```python
from build123d import *

# Parameters (mm, degrees)
ESQUISSE1_R          = 0.6
BASE_EXTRUSION_DEPTH = 1


with BuildPart() as part:
    # Esquisse1 → Base-Extrusion (new body)
    with BuildSketch(Plane.XY):
        with BuildLine():
            Line((-4.406978672, 11.661475663), (-4.564568548, 12.078480291))
            ThreePointArc((-4.564568548, 12.078480291), (-5.131923481, 12.654767663), (-5.94, 12.622969933))
            ThreePointArc((-5.94, 12.622969933), (0, -13), (5.94, 12.622969933))
            ThreePointArc((5.94, 12.622969933), (5.131923481, 12.654767663), (4.564568548, 12.078480291))
            Line((4.564568548, 12.078480291), (4.406978672, 11.661475663))
            ThreePointArc((4.406978672, 11.661475663), (2.882284348, 12.148709668), (1.306307585, 12.428686453))
            Line((1.306307585, 12.428686453), (1.567926949, 14.917828431))
            ThreePointArc((1.567926949, 14.917828431), (0, -15), (-1.567926949, 14.917828431))
            Line((-1.567926949, 14.917828431), (-1.306307585, 12.428686453))
            ThreePointArc((-1.306307585, 12.428686453), (-2.882284348, 12.148709668), (-4.406978672, 11.661475663))
        make_face()
        with Locations((-3, 13.4)):
            Circle(ESQUISSE1_R, mode=Mode.SUBTRACT)
        with Locations(Location((3, 13.4, 0), (0, 0, 180))):
            Circle(ESQUISSE1_R, mode=Mode.SUBTRACT)
    extrude(amount=BASE_EXTRUSION_DEPTH)


solid = part.part
```
Check sheet for the modelled part. Datum: model origin and axes. Units: mm. A direction names the side the tool comes from. Coordinates: 2 decimals unless noted, no trailing zeros. Loops run counter-clockwise (first coordinate to the right, second up) from the corner with the lowest first, then second, coordinate; pieces in that order, holes last.
1) Release check for a two-part mould opening along X. For faces 4 (the face through (5.14, 12.66, 0.49)), 5 (the face through (0.1, -13.3, 1)), 6 (the face through (0.638, -14.986, 0.493)) record: released by +X, released by -X, zero draft, split by the parting line, or undercut.
2) Sectioned sample at D-D (x = -9.5). Record the boundary of the cut face in (y, z), and give its area (3 significant figures).
3) Sectioned sample at C-C (x = 3). Record the boundary of the cut face in (y, z), and give its area (3 significant figures).
4) Access from +Z, -Z, +X, -X, +Y, -Y to the whole of each face (thin tool, end or side, straight path). Record for faces 1 (the face through (1.435, 13.656, 0.493)), 2 (the face through (0.1, -13.3, 0)), 3 (the face through (2.904, 12.143, 0.493)).
5) Sectioned sample at B-B (y = 8.25). Record the boundary of the cut face in (x, z).
6) Sectioned sample at A-A (z = 0.5). Record the boundary of the cut face in (x, y), and give its area (3 significant figures).
7) Gauge pin test, flat end, axial feed: pin 1 (1.4 mm diameter, centred on x = 3, y = 13.4, fed in from +Z). Record the tip position at first contact, or that the pin passes through.
8) Material ranges on probe 1 along Y at (x, z) = (3, 0.6); probe 2 along Y at (x, z) = (3.5, 0.15); probe 3 along X at (y, z) = (0.5, 0.65), recorded low to high.
Check sheet entries:
1. face 4: undercut
1. face 5: zero draft
1. face 6: split by the parting line
2. outline: (-11.61, 0) - (-9.09, 0) - (-9.09, 1) - (-11.61, 1) - close; (10.09, 0) - (11.61, 0) - (11.61, 1) - (10.09, 1) - close
2. area: 4.03 mm2
3. outline: (-14.7, 0) - (-12.66, 0) - (-12.66, 1) - (-14.7, 1) - close; (12.12, 0) - (12.8, 0) - (12.8, 1) - (12.12, 1) - close; (14, 0) - (14.7, 0) - (14.7, 1) - (14, 1) - close
3. area: 3.41 mm2
4. face 1: +Z, -Z, +Y
4. face 2: -Z, +X, -X, +Y, -Y
4. face 3: +Z, -Z
5. outline: (-12.53, 0) - (-11.05, 0) - (-11.05, 1) - (-12.53, 1) - close; (11.05, 0) - (12.53, 0) - (12.53, 1) - (11.05, 1) - close
6. outline: (-5.94, 12.62) arc R1 cw to (-4.56, 12.08) - (-4.41, 11.66) arc R12 cw to (-1.31, 12.43) - (-1.57, 14.92) arc R15 ccw (long way) to (1.57, 14.92) - (1.31, 12.43) arc R12 cw to (4.41, 11.66) - (4.56, 12.08) arc R1 cw to (5.94, 12.62) arc R13.5 cw (long way) to start; hole circle Ø1.2 at (-3, 13.4); hole circle Ø1.2 at (3, 13.4)
6. area: 140 mm2
7. pin 1: stops at z = 1
8. probe 1: y = -14.7 to -12.66, 12.12 to 12.8, 14 to 14.7
8. probe 2: y = -14.59 to -12.54, 11.98 to 13.07, 13.73 to 14.59
8. probe 3: x = -14.99 to -13.5, 13.5 to 14.99
